from build123d import *

# Parameters (mm, degrees)
SHELL1_T              = -2.54
SKETCH5_R             = 3.175
SKETCH5_R_2           = 1.905
BOSS_EXTRUDE1_DEPTH   = 15.24
BOSS_EXTRUDE1_2_DEPTH = 15.24
CUT_EXTRUDE1_REACH    = 31.116
SKETCH6_R             = 3.392080707
SKETCH7_R             = 10.16
SKETCH7_R_2           = 3.175
BOSS_EXTRUDE2_DEPTH   = 2.54


with BuildPart() as part:
    # Sketch4 → Revolve1 (revolve)
    with BuildSketch(Plane(origin=(0, 0, 0), x_dir=(0, 0, -1), z_dir=(1, 0, 0))):
        Polygon((0, 0), (-3.392080707, 0), (-10.16, 2.463321171), (-10.16, 10.083321171), (0, 10.083321171), align=None)
    revolve(axis=Axis((0, 10.083321171, 0), (0, -1, 0)))

    # Shell1
    shell1_openings = [part.faces().sort_by_distance(p)[0] for p in [
        (0, 10.083321171, 0),
    ]]
    offset(amount=SHELL1_T, openings=shell1_openings, kind=Kind.INTERSECTION)

    # Cut-Extrude1: up to this cone (the profile starts outside it)
    cut_extrude1_end = Plane(origin=(0, 0, 0), z_dir=(0, 1, 0)).offset(1.468396133) * Cone(2.747e-06, 82.829863624, 30.147603867, align=(Align.CENTER, Align.CENTER, Align.MIN), mode=Mode.PRIVATE)
    # Sketch6 → Cut-Extrude1 (cut, up to the surface)
    with BuildSketch(Plane.XZ, mode=Mode.PRIVATE) as cut_extrude1_sk1:
        with Locations(Location((0, 0, 0), (0, 0, 90))):
            Circle(SKETCH6_R)
    cut_extrude1_tool1 = extrude(cut_extrude1_sk1.sketch, amount=-CUT_EXTRUDE1_REACH, mode=Mode.PRIVATE) - cut_extrude1_end
    add(cut_extrude1_tool1.solids().sort_by_distance((0, 0, 0))[0], mode=Mode.SUBTRACT)


with BuildPart() as body_2:
    # Sketch5 → Boss-Extrude1 (new body)
    with BuildSketch(Plane(origin=(0, 10.083321171, 0), x_dir=(1, 0, 0), z_dir=(0, 1, 0))):
        with Locations(Location((-4.318, 0, 0), (0, 0, 90))):
            Circle(SKETCH5_R)
        with Locations(Location((-4.318, 0, 0), (0, 0, 90))):
            Circle(SKETCH5_R_2, mode=Mode.SUBTRACT)
    extrude(amount=BOSS_EXTRUDE1_DEPTH)



with BuildPart() as body_3:
    # Sketch5 → Boss-Extrude1 2 (new body)
    with BuildSketch(Plane(origin=(0, 10.083321171, 0), x_dir=(1, 0, 0), z_dir=(0, 1, 0))):
        with Locations(Location((4.318, 0, 0), (0, 0, 90))):
            Circle(SKETCH5_R)
        with Locations(Location((4.318, 0, 0), (0, 0, 90))):
            Circle(SKETCH5_R_2, mode=Mode.SUBTRACT)
    extrude(amount=BOSS_EXTRUDE1_2_DEPTH)


with BuildPart() as cut_extrude1_kept_piece:
    # of the separate pieces the step leaves, the one the design keeps (cut_extrude1_pieces_kept)
    add(part.part.solids().sort_by_distance((0, 0, 3.392080707))[0])


with BuildPart() as body_2_1:
    add(body_2.part)

    add(body_3.part)  # Boss-Extrude2 merges body 3

    add(cut_extrude1_kept_piece.part)  # Boss-Extrude2 merges Cut-Extrude1 kept piece
    # Sketch7 → Boss-Extrude2 (add)
    with BuildSketch(Plane(origin=(0, 10.083321171, 0), x_dir=(1, 0, 0), z_dir=(0, 1, 0))):
        with Locations(Location((0, 0, 0), (0, 0, 270))):
            Circle(SKETCH7_R)
        with Locations(Location((-4.318, 0, 0), (0, 0, 90))):
            Circle(SKETCH7_R_2, mode=Mode.SUBTRACT)
        with Locations(Location((4.318, 0, 0), (0, 0, 90))):
            Circle(SKETCH7_R_2, mode=Mode.SUBTRACT)
    extrude(amount=BOSS_EXTRUDE2_DEPTH)


solid = body_2_1.part
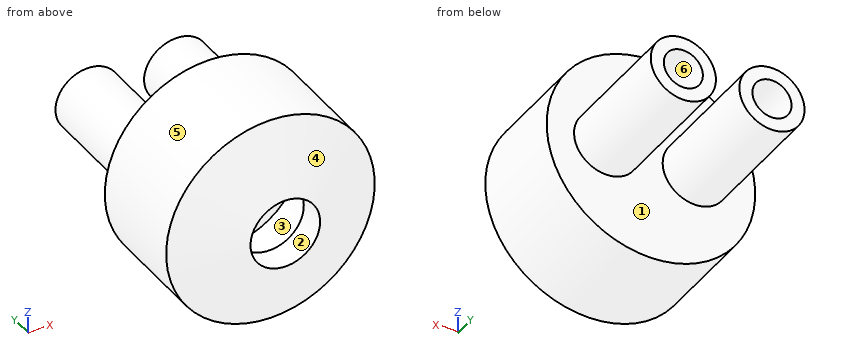
Verification items for the finished model (mm, model axes). Face numbers are marked on the shaded views. A direction names the side the tool comes from. Give positions to 0.01 mm unless a question says otherwise; leave off trailing zeros. Loops run counter-clockwise (first coordinate to the right, second up) from the corner with the lowest first, then second, coordinate; pieces in that order, holes last.
1) Sectioned sample at D-D, the plane y = 6. Enter the section's corners in (x, z).
2) Sectioned sample at A-A, the plane z = 0. Enter the section's corners in (x, y), then the cut area to 3 significant figures.
3) Draft check along Z on the marked faces 1, 2, 3 and 4. Enter one of: pulls with the +Z half, pulls with the -Z half, needs draft (parallel to the pull), parting line crosses it, or undercut.
4) Thickness scan on line 1 along X through (y, z) = (13, 0); line 2 along Z through (x, y) = (4.25, 12.75); line 3 along Z through (x, y) = (-5.5, 17.5). Record the ranges inside material, lowest first.
5) Sectioned sample at B-B, the plane y = 18.25. Enter the section's corners in (x, z) (3 decimals), then the cut area to 3 significant figures.
6) Depth check by flat-ended pin: pin 1 Ø8 at (x, y) = (-5, 8) entering from -Z; pin 2 Ø5 at (x, y) = (5.5, 18.5) entering from -Z (3 decimals); pin 3 Ø8 at (y, z) = (9, 7) entering from -X. Enter the tip coordinate at first touch or a pass-through.
7) Sectioned sample at C-C, the plane x = 0. Enter the section's corners in (y, z), then the cut area to 3 significant figures.
8) Set-up check for the marked faces 5 and 6: record each of +Z, -Z, +X, -X, +Y, -Y from which the full face is reachable in a straight line by a thin tool's end or side.
Answers:
1. outline: circle Ø20.32 at (0, 0); hole circle Ø15.24 at (0, 0)
2. outline: (-10.16, 2.46) - (-3.39, 0) - (-3.39, 2.7) - (-7.62, 4.24) - (-7.62, 10.08) - (-6.22, 10.08) - (-6.22, 25.32) - (-7.49, 25.32) - (-7.49, 12.62) - (-10.16, 12.62) - close; (-2.41, 10.08) - (2.41, 10.08) - (2.41, 25.32) - (1.14, 25.32) - (1.14, 12.62) - (-1.14, 12.62) - (-1.14, 25.32) - (-2.41, 25.32) - close; (3.39, 0) - (10.16, 2.46) - (10.16, 12.62) - (7.49, 12.62) - (7.49, 25.32) - (6.22, 25.32) - (6.22, 10.08) - (7.62, 10.08) - (7.62, 4.24) - (3.39, 2.7) - close
2. area: 161 mm2
3. face 1: needs draft
3. face 2: undercut
3. face 3: undercut
3. face 4: parting line crosses it
4. line 1: x = -7.49 to -6.22, -2.41 to -1.14, 1.14 to 2.41, 6.22 to 7.49
4. line 2: z = -3.17 to -1.9, 1.9 to 3.17
4. line 3: z = -2.95 to -1.49, 1.49 to 2.95
5. outline: circle Ø6.35 at (-4.318, 0); circle Ø6.35 at (4.318, 0); hole circle Ø3.81 at (-4.318, 0); hole circle Ø3.81 at (4.318, 0)
5. area: 40.5 mm2
6. pin 1: stops at z = -10.11
6. pin 2: stops at z = -3.175
6. pin 3: stops at x = -9.71
7. outline: (0, -3.39) - (2.46, -10.16) - (12.62, -10.16) - (12.62, 10.16) - (2.46, 10.16) - (0, 3.39) - (2.7, 3.39) - (4.24, 7.62) - (10.08, 7.62) - (10.08, -7.62) - (4.24, -7.62) - (2.7, -3.39) - close
7. area: 116 mm2
8. face 5: +Y, -Y
8. face 6: +Y
